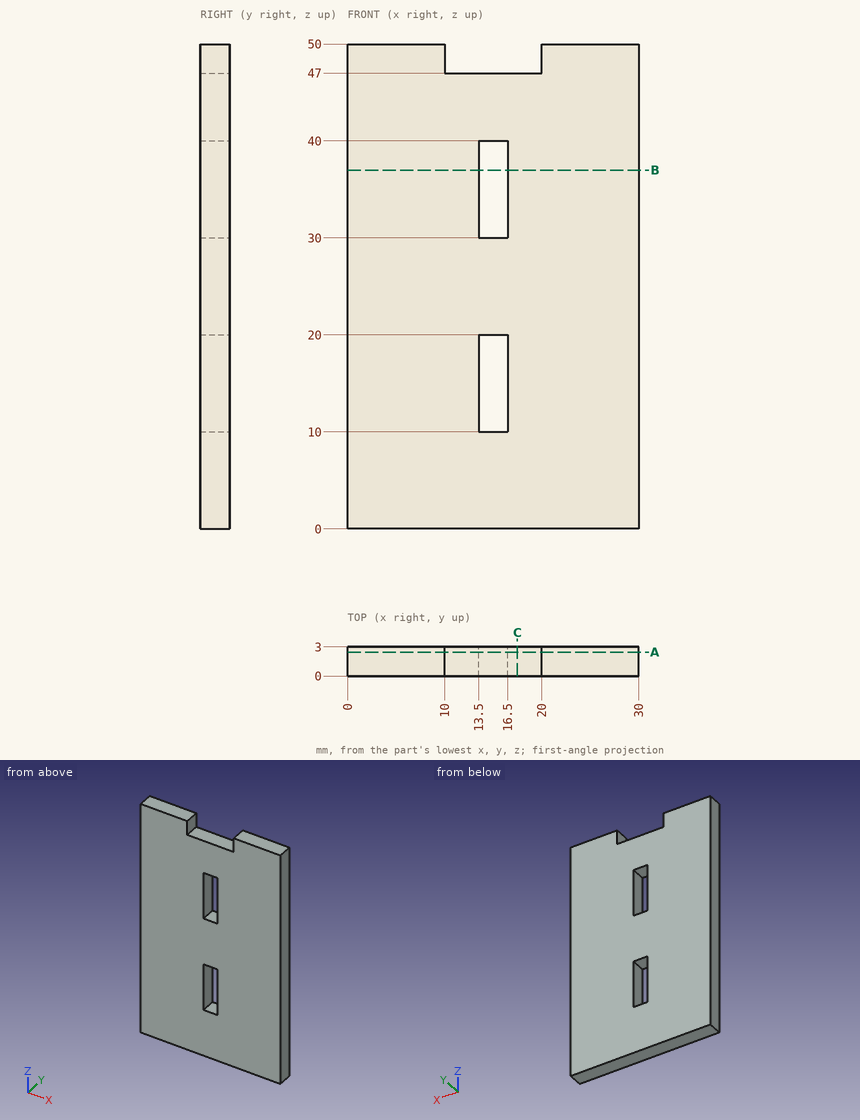
Source: three-view drawing plus pictorial views. Frame: mm from the lowest corner of the part. Round coordinates to 2 decimals unless told otherwise and drop trailing zeros. Write each loop counter-clockwise with the first axis right and the second up, starting at its lowest first coordinate (ties: lowest second). Pieces come first, ordered by that corner, then holes. Notation, with made-up numbers: M 77,35 L 81,35 A13 ccw 81,46 Z; hole C 71.25,-33 d8. An arc over 180 degrees is marked long. Write each question's results on one line, items separated by ' | '.
Q1. Section query A-A (y = 2.45). Return loops of the section in (x, z).
Results:
outline: M 0,0 L 30,0 L 30,50 L 20,50 L 20,47 L 10,47 L 10,50 L 0,50 Z; hole M 13.5,10 L 16.5,10 L 16.5,20 L 13.5,20 Z; hole M 13.5,30 L 16.5,30 L 16.5,40 L 13.5,40 Z
Q2. Pin query (flat end, axial travel): P1, Ø1.5, axis at x = 15.5, y = 1.5, coming from the +Z side. Return the tip coordinate at first contact, or that it passes through.
Results:
P1: stops at z = 47
Q3. Section query B-B (z = 37). Return loops of the section in (x, y).
Results:
outline: M 0,0 L 13.5,0 L 13.5,3 L 0,3 Z; M 16.5,0 L 30,0 L 30,3 L 16.5,3 Z
Q4. Section query C-C (x = 17.5). Return loops of the section in (y, z).
Results:
outline: M 0,0 L 3,0 L 3,47 L 0,47 Z
Q5. Line query: line 1 along X through (y, z) = (0.95, 30.5); line 2 along Z through (x, y) = (12, 2.3). Output: solid intervals per line, ascending.
Results:
line 1: x = 0 to 13.5, 16.5 to 30 | line 2: z = 0 to 47
